Autodesk Inventor part; units mm, degrees
ref_plane "YZ Plane" through (0, 0, 0) normal (1, 0, 0) x (0, 1, 0)
ref_plane "XZ Plane" through (0, 0, 0) normal (0, 1, 0) x (-1, 0, 0)
ref_plane "XY Plane" through (0, 0, 0) normal (0, 0, 1) x (1, 0, 0)
sketch "Skizze1" plane through (0, 0, 0) normal (0, 1, 0) x (-1, 0, 0)
  circle A0 centre (0, 0) radius 20
  dimension "d0" = 40
extrude "Extrusion1" add sketch "Skizze1" along normal blind 26
ref_plane "Arbeitsebene1" through (0, 26, 0) normal (0, 1, 0) x (1, 0, 0)
sketch "Skizze2" plane through (0, 26, 0) normal (0, 1, 0) x (1, 0, 0)
  circle A0 centre (0, 0) radius 20
  circle A1 centre (0, 0) radius 20 construction
  circle A2 centre (0, 0) radius 20 construction
  line L0 (-15, 0) -> (15, 0) construction
  dimension "d42" = 15
  dimension "d43" = 15
ref_plane "Arbeitsebene2" through (0, 0, 0) normal (0, -1, 0) x (1, 0, 0)
sketch "Skizze3" plane through (0, 0, 0) normal (0, -1, 0) x (1, 0, 0)
  circle A0 centre (0, 0) radius 20
hole "Bohrung2" at (0, 0, 0) direction (0, 1, 0) diameter 6 depth 20
sketch "Skizze4" plane through (0, 0, 0) normal (0, -1, 0) x (1, 0, 0)
  point P0 (0, 0)
sketch "Skizze5" plane through (0, 0, 0) normal (0, -1, 0) x (1, 0, 0)
  line L0 (0, 0) -> (0, 20) construction
  circle A0 centre (0, 0) radius 20 construction
ref_plane "Arbeitsebene3" through (0, 0, 20) normal (0, 0, 1) x (1, 0, 0)
sketch "Skizze6" plane through (0, 0, 20) normal (0, 0, 1) x (1, 0, 0)
  line L0 (0, 0) -> (0, 27.6738) construction
  point P0 (0, 8)
  point P1 (0, 16)
  dimension "d25" = 8
  dimension "d26" = 8
hole "Bohrung3" at (0, 16, 20) at (0, 8, 20) direction (0, 0, -1) diameter 3 depth 20 tip angle 118
sketch "Skizze7" plane through (0, 0, 0) normal (0, -1, 0) x (1, 0, 0)
  circle A0 centre (0, 0) radius 6.5
  circle A1 centre (0, 0) radius 20
  dimension "d38" = 13
  dimension "d39" = 40
extrude "Extrusion2" cut sketch "Skizze7" against normal blind 20
hole "Bohrung4" at (-15, 26, 0) at (15, 26, 0) direction (0, -1, 0) diameter 4 end through all
sketch "Skizze8" plane through (0, 0, 0) normal (0, -1, 0) x (1, 0, 0)
  line L0 (-20, 7.5) -> (20, 7.5)
  line L1 (20, 7.5) -> (20, -7.5)
  line L2 (20, -7.5) -> (-20, -7.5)
  line L3 (-20, -7.5) -> (-20, 7.5)
  line L4 (-20, 7.5) -> (20, -7.5) construction
  line L5 (20, 7.5) -> (-20, -7.5) construction
  point P0 (0, 0)
  dimension "d52" = 40
  dimension "d53" = 15
extrude "Extrusion3" cut sketch "Skizze8" against normal through all keep common part
sketch "Skizze9" plane through (0, 0, 0) normal (0, -1, 0) x (1, 0, 0)
  line L0 (-15, -15) -> (15, -15)
  line L1 (15, -15) -> (15, 15)
  line L2 (15, 15) -> (-15, 15)
  line L3 (-15, 15) -> (-15, -15)
  line L4 (-15, -15) -> (15, 15) construction
  line L5 (15, -15) -> (-15, 15) construction
  point P0 (0, 0)
  dimension "d56" = 30
  dimension "d57" = 30
extrude "Extrusion4" cut sketch "Skizze9" against normal blind 3
thread "Gewinde5"
thread "Gewinde6"
thread "Gewinde7"
thread "Gewinde8"
sketch "Skizze10" plane through (0, 26, 0) normal (0, 1, 0) x (1, 0, 0)
  arc A0 (-18.5405, 7.5) -> (-18.5405, -7.5) centre (0, 0) ccw
  line L0 (18.5405, 7.5) -> (-18.5405, 7.5)
  line L1 (-18.5405, 7.5) -> (-18.5405, -7.5)
  line L2 (-18.5405, -7.5) -> (18.5405, -7.5)
  line L3 (18.5405, -7.5) -> (18.5405, 7.5)
  line L4 (18.5405, 7.5) -> (-18.5405, -7.5) construction
  line L5 (-18.5405, 7.5) -> (18.5405, -7.5) construction
extrude "Extrusion5" cut sketch "Skizze10" against normal through all contours L0 L3 L2 L1 keep common part
fillet "Rundung1" radius 2 4 edges at (18.5405, 23, -7.5) (18.5405, 23, 7.5) (-18.5405, 23, -7.5) (-18.5405, 23, 7.5)
thread "Gewinde9"
thread "Gewinde10"
thread "Gewinde11"
thread "Gewinde12"
properties part number "spannring_achse"
The model under review builds one solid part; all positions refer to its coordinate system, in mm. A direction names the side the tool comes from. Round coordinates to 2 decimals unless told otherwise and drop trailing zeros. Write each loop counter-clockwise with the first axis right and the second up, starting at its lowest first coordinate (ties: lowest second). Pieces come first, ordered by that corner, then holes. Notation, with made-up numbers: (50.5, -28) - (107.5, -28) arc R14 ccw to (107.5, -11) - close; hole circle Ø1 at (61, -4). An arc over 180 degrees is marked (long way). One line per question, with ' | ' between items.
Item 1: To check wall thickness, follow probe 1 along X at (y, z) = (23.7, 0); probe 2 along Z at (x, y) = (15, 23.1); probe 3 along Z at (x, y) = (0, 13.25). State the ranges of each line that lie inside material, in increasing order.
Resolved:
probe 1: x = -18.54 to -17, -13 to 13, 17 to 18.54 | probe 2: z = -7.5 to -2, 2 to 7.5 | probe 3: z = -6.5 to -3, 3 to 6.5
Item 2: Add section D-D, the plane z = 4. Give the boundary of the cut face in (x, y), then the cut area to 3 significant figures.
Resolved:
outline: (-18.54, 20) - (-5.12, 20) - (-5.12, 3) - (5.12, 3) - (5.12, 20) - (18.54, 20) - (18.54, 26) - (-18.54, 26) - close; hole circle Ø3 at (0, 8); hole circle Ø3 at (0, 16) | area: 383 mm2
Item 3: Add section A-A, the plane x = 0. Give the boundary of the cut face in (y, z).
Resolved:
outline: (3, -6.5) - (20, -6.5) - (20, -7.5) - (26, -7.5) - (26, 7.5) - (20, 7.5) - (20, 6.5) - (17.5, 6.5) - (17.5, 3) - (20, 3) - (20, -3) - (3, -3) - close; (3, 3) - (6.5, 3) - (6.5, 6.5) - (3, 6.5) - close; (9.5, 3) - (14.5, 3) - (14.5, 6.5) - (9.5, 6.5) - close
Item 4: For P1, Ø3, axis at y = 12, z = 0, coming from the +X side; P2, Ø1.8, axis at x = 0, y = 16, coming from the +Z side; P3, Ø12, axis at x = -10.5, y = 6, coming from the +Z side; P4, Ø3, axis at x = -15, z = 0, coming from the +Y side, all flat-tipped, find the tip position at first contact; note any pin that passes through.
Resolved:
P1: stops at x = 6.5 | P2: stops at z = -2.86 | P3: stops at z = 4.69 | P4: passes through
Item 5: Add section B-B, the plane x = 15. Give the boundary of the cut face in (y, z), then the cut area to 3 significant figures.
Resolved:
outline: (20, -7.5) - (26, -7.5) - (26, -2) - (20, -2) - close; (20, 2) - (26, 2) - (26, 7.5) - (20, 7.5) - close | area: 66.0 mm2
Item 6: For faces 1 (the face through (0.575, 6.614, 4.522)), 2 (the face through (18.54, 23, 0)), 3 (the face through (-0.9, 11.62, -2.86)), list the 3-axis set-ups (+Z, -Z, +X, -X, +Y, -Y) from which the entire face can be reached by the end or side of a thin tool; tool diameter is ignored.
Resolved:
face 1: +Z | face 2: +Z, -Z, +X, +Y, -Y | face 3: -Y
Item 7: The part is to be moulded in two halves that separate along Z. For faces 4 (the face through (0, 26, 0)), 5 (the face through (13, 23, 0)), 6 (the face through (0, 23, 7.5)), say which applies: pulls with the +Z half, pulls with the -Z half, needs draft (parallel to the pull), parting line crosses it, or undercut.
Resolved:
face 4: needs draft | face 5: undercut | face 6: pulls with the +Z half
Item 8: Add section C-C, the plane y = 22.5. Give the boundary of the cut face in (x, z), then the cut area to 3 significant figures.
Resolved:
outline: (-18.54, -5.5) arc R2 ccw to (-16.54, -7.5) - (16.54, -7.5) arc R2 ccw to (18.54, -5.5) - (18.54, 5.5) arc R2 ccw to (16.54, 7.5) - (-16.54, 7.5) arc R2 ccw to (-18.54, 5.5) - close; hole circle Ø4 at (-15, 0); hole circle Ø4 at (15, 0) | area: 528 mm2
